Autodesk Inventor part; units mm, degrees
ref_plane "YZ Plane" through (0, 0, 0) normal (1, 0, 0) x (0, 1, 0)
ref_plane "XZ Plane" through (0, 0, 0) normal (0, 1, 0) x (-1, 0, 0)
ref_plane "XY Plane" through (0, 0, 0) normal (0, 0, 1) x (1, 0, 0)
sketch "Esboço1" plane through (0, 0, 0) normal (1, 0, 0) x (0, 1, 0)
  line L0 (8.7685, 9.8534) -> (4.4419, 3.3376)
  line L1 (4.4419, 3.3376) -> (1.0821, 5.5685)
  line L2 (1.0821, 5.5685) -> (3.8705, 9.768)
  line L3 (-5.1511, 5.9928) -> (0.9304, 2.875)
  line L4 (0.9304, 2.875) -> (-3.5768, -6.1466)
  line L5 (8.7685, 9.8534) -> (8.7685, -5.5484)
  line L6 (8.7685, -5.5484) -> (-3.5905, -6.174)
  line L7 (-3.5905, -6.174) -> (-3.5768, -6.1466)
  arc A0 (-5.1511, 5.9928) -> (3.8705, 9.768) centre (-3.4697, 14.6419) ccw
extrude "Extrusão1" add sketch "Esboço1" along normal blind 330
properties part number "juncao tela - som"
CAD build for the part. Positions are in the model's coordinates, mm. A direction names the side the tool comes from. Round coordinates to 2 decimals unless told otherwise and drop trailing zeros.
(1) Probe line 1 along Y through (x, z) = (215, 6.5); line 2 along Y through (x, z) = (103, 5); line 3 along Z through (x, y) = (78, -0.25). List the from-to ranges inside material, lowest first.
(2) Mould opens along Z. For faces 3 (the face through (162.69, -0.002, 6.542)), 4 (the face through (0, 3, 0)), 5 (the face through (162.69, -2.153, 4.456)) say: pulls with the +Z half, pulls with the -Z half, needs draft (parallel to the pull), parting line crosses it, or undercut.
(3) 3-axis set-ups, long thin cutter, end or side, ignore diameter. For faces 1 (the face through (330, 3, 0)), 2 (the face through (162.69, 6.635, 6.641)): which of +Z, -Z, +X, -X, +Y, -Y reach the whole face in a straight line?
(4) Drop flat-ended pins along their axis: P1, Ø6, axis at x = 186.5, y = 4, coming from the -Z side; P2, Ø5, axis at x = 267, y = -0.5, coming from the +Z side; P3, Ø4, axis at x = 166.5, z = 5.5, coming from the -Y side. Give the stop position or say it passes through.
From the geometry:
1. line 1: y = -0.1 to 1.7, 6.54 to 8.77
1. line 2: y = -3.21 to 1.94, 5.55 to 8.77
1. line 3: z = -6 to 0.51, 3.48 to 6.44
2. face 3: pulls with the +Z half
2. face 4: needs draft
2. face 5: undercut
3. face 1: +Z, -Z, +X, +Y, -Y
3. face 2: +Z, +X, -X
4. P1: stops at z = -5.94
4. P2: stops at z = 7.73
4. P3: stops at y = -5.15
